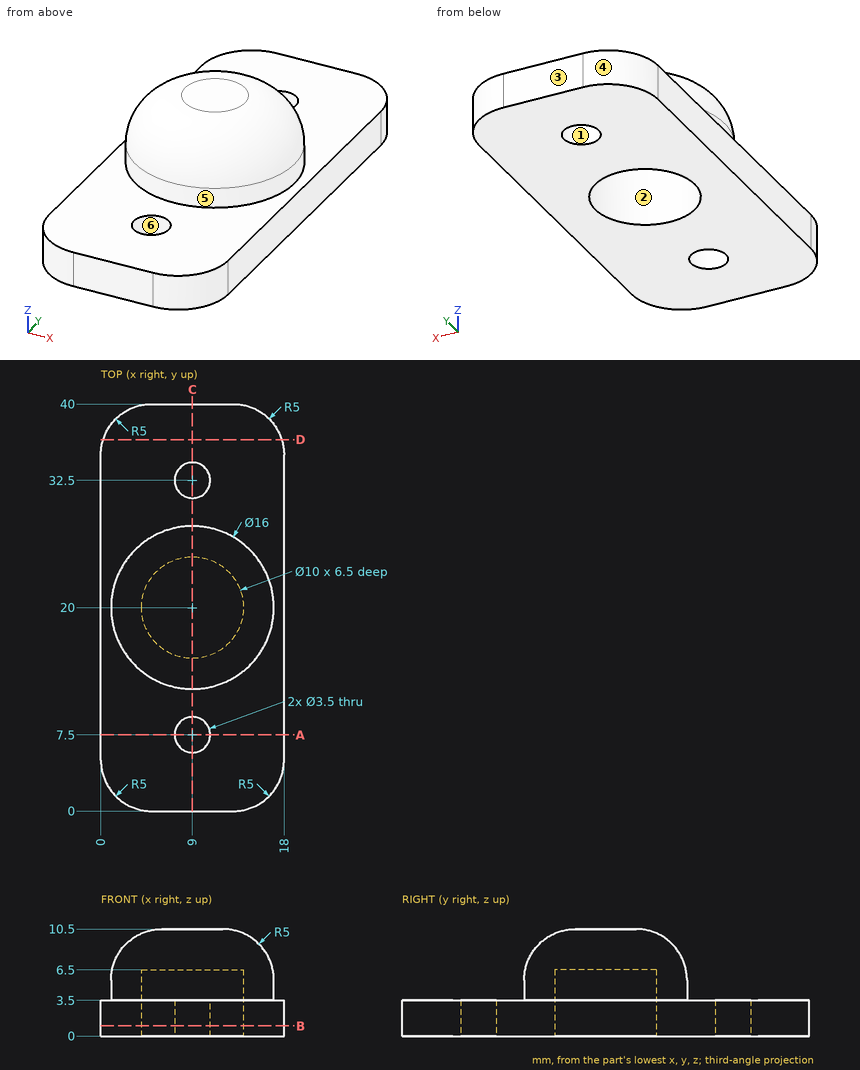
Job drawing, mm, ordinate dimensions from the low corner. One solid piece. A direction names the side the tool comes from. Coordinates: 2 decimals unless noted, no trailing zeros. Order: outer loops, then holes, each group sorted by start corner. A loop starts at its lowest first (then second) coordinate and runs counter-clockwise, first axis right, second up. Notation, with made-up numbers: (-33.75, 63) -> (25.25, 63) arc R20 ccw to (25.25, 74) -> close; hole circle Ø8 at (76.25, -8.5). An arc over 180 degrees is marked (long way). Answer in a Markdown table with one row per item. Add a question column.
Q1. Band-saw the part on A-A, the plane y = 7.5. List the corners of the cut face in (x, z), then the cut area to 4 significant figures.
Q2. Mould opens along X. For the marked faces 3, 4, 5 and 6 say: +X half, -X half, draft (parallel to the pull), parting line (faces both ways), or undercut.
Q3. Drop flat-ended pins along their axis: pin 1 (3 mm diameter, centred on x = 13, y = 4.5, fed in from +Z); pin 2 (9 mm diameter, centred on x = 13, y = 29, fed in from +Z); pin 3 (1 mm diameter, centred on x = 3, z = 2, fed in from +Y). Give the stop position or say it passes through.
Q4. Band-saw the part on D-D, the plane y = 36.5. List the corners of the cut face in (x, z), then the cut area to 3 significant figures.
Q5. Which spindle directions (+Z, -Z, +X, -X, +Y, -Y) get a long thin tool onto all of the face, cutting with end or side? Do the marked faces 1 and 2. Say none if no direction does.
Q6. Band-saw the part on B-B, the plane z = 1. List the corners of the cut face in (x, y), then the cut area to 3 significant figures.
Q7. Wall check: line 1 along Y through (x, z) = (9, 1.2); line 2 along Y through (x, z) = (10.5, 1.75); line 3 along Z through (x, y) = (3.5, 8). Give the ranges that are in metal, low to high. Write a range as [from, to].
Q8. Band-saw the part on C-C, the plane x = 9. Give the number of separate pieces and of enclosed holes in the cut face, then the cut area to 3 significant figures.
Answers follow:
| question | item | result |
|---|---|---|
| 1 | outline | (0, 0) -> (7.25, 0) -> (7.25, 3.5) -> (0, 3.5) -> close; (10.75, 0) -> (18, 0) -> (18, 3.5) -> (10.75, 3.5) -> close |
| 1 | area | 50.75 mm^2 |
| 2 | face 3 | draft |
| 2 | face 4 | -X half |
| 2 | face 5 | parting line |
| 2 | face 6 | undercut |
| 3 | pin 1 | z = 3.5 |
| 3 | pin 2 | z = 9.91 |
| 3 | pin 3 | y = 39.77 |
| 4 | outline | (0.23, 0) -> (17.77, 0) -> (17.77, 3.5) -> (0.23, 3.5) -> close |
| 4 | area | 61.4 mm^2 |
| 5 | face 1 | +Z, -Z |
| 5 | face 2 | -Z |
| 6 | outline | (0, 5) arc R5 ccw to (5, 0) -> (13, 0) arc R5 ccw to (18, 5) -> (18, 35) arc R5 ccw to (13, 40) -> (5, 40) arc R5 ccw to (0, 35) -> close; hole circle Ø10 at (9, 20); hole circle Ø3.5 at (9, 7.5); hole circle Ø3.5 at (9, 32.5) |
| 6 | area | 601 mm^2 |
| 7 | line 1 | [0, 5.75], [9.25, 15], [25, 30.75], [34.25, 40] |
| 7 | line 2 | [0, 6.6], [8.4, 15.23], [24.77, 31.6], [33.4, 40] |
| 7 | line 3 | [0, 3.5] |
| 8 | separate pieces | 3 |
| 8 | enclosed holes | 0 |
| 8 | area | 152 mm^2 |
